The model under review builds one solid part; all positions refer to its coordinate system, in mm. Face numbers are marked on the shaded views. A direction names the side the tool comes from. Coordinates: 2 decimals unless noted, no trailing zeros. Write each loop counter-clockwise with the first axis right and the second up, starting at its lowest first coordinate (ties: lowest second). Pieces come first, ordered by that corner, then holes. Notation, with made-up numbers: M -2.75,83.25 L 48.25,83.25 A21 ccw 48.25,122.25 Z; hole C 25.25,22 d9. An arc over 180 degrees is marked long. Answer as CSV lines item,"result". Start each with the question number.
from build123d import *

# Parameters (mm, degrees)
PAD005_DEPTH           = 1
SKETCH011_R            = 2.05
POCKET008_DEPTH        = 0.32
LINEARPATTERN002_COUNT = 2
LINEARPATTERN002_PITCH = 8.7
LINEARPATTERN003_COUNT = 2
LINEARPATTERN003_PITCH = 8.7
SKETCH013_W            = 3
SKETCH013_H            = 0.75
POCKET009_DEPTH        = 0.5


with BuildPart() as part:
    # Sketch010 (on DatumPlane) → Pad005 (new body)
    with BuildSketch(Plane(origin=(0, 0, 1.2), x_dir=(1, 0, 0), z_dir=(0, 0, -1))):
        with BuildLine():
            ThreePointArc((18.55, -6.11), (14.55, -10.11), (18.55, -14.11))
            Line((18.55, -14.11), (27.25, -14.11))
            ThreePointArc((27.25, -14.11), (31.25, -10.11), (27.25, -6.11))
            Line((18.55, -6.11), (27.25, -6.11))
        make_face()
    extrude(amount=-PAD005_DEPTH)

    # Sketch011 (on Face2 of Pad005) → Pocket008 (cut)
    with BuildSketch(Plane(origin=(0, 0, 1.2), x_dir=(1, 0, 0), z_dir=(0, 0, -1))):
        with Locations((18.55, -10.11)):
            Circle(SKETCH011_R)
    pocket008 = extrude(amount=-POCKET008_DEPTH, mode=Mode.SUBTRACT)

    # LinearPattern002: Pocket008 ×2
    with Locations(*[(i * LINEARPATTERN002_PITCH, 0, 0) for i in range(1, LINEARPATTERN002_COUNT)]):
        add(pocket008, mode=Mode.SUBTRACT)

    # Sketch012 (on DatumPlane) → Revolution001 (revolve)
    with BuildSketch(Plane(origin=(18.55, 6.74, 1.2), x_dir=(0, -1, 0), z_dir=(-1, 0, 0))):
        with BuildLine():
            Line((-3.37, 1), (-3.37, 2.4))
            ThreePointArc((-0.604564, 2.25), (-1.985249, 2.362472), (-3.37, 2.4))
            ThreePointArc((-0.47, 2.1), (-0.508571, 2.200756), (-0.604564, 2.25))
            Line((-0.47, 1), (-0.47, 2.1))
            Line((-3.37, 1), (-0.47, 1))
        make_face()
    revolution001 = revolve(axis=Axis((18.55, 10.11, 1.2), (0, 0, -1)))

    # LinearPattern003: Revolution001 ×2
    with Locations(*[(i * LINEARPATTERN003_PITCH, 0, 0) for i in range(1, LINEARPATTERN003_COUNT)]):
        add(revolution001)

    # Sketch013 (on DatumPlane) → Pocket009 (cut)
    with BuildSketch(Plane(origin=(27.25, 10.11, 3.6), x_dir=(-1, 0, 0), z_dir=(0, 0, 1))):
        Polygon((1, 1.732051), (-2, 0), (1, -1.732051), align=None)
        with Locations((8.7, 0)):
            Rectangle(SKETCH013_W, SKETCH013_H)
        with Locations((8.7, 1.125)):
            Rectangle(SKETCH013_W, SKETCH013_H)
        with Locations((8.7, -1.125)):
            Rectangle(SKETCH013_W, SKETCH013_H)
    extrude(amount=-POCKET009_DEPTH, mode=Mode.SUBTRACT)


solid = part.part
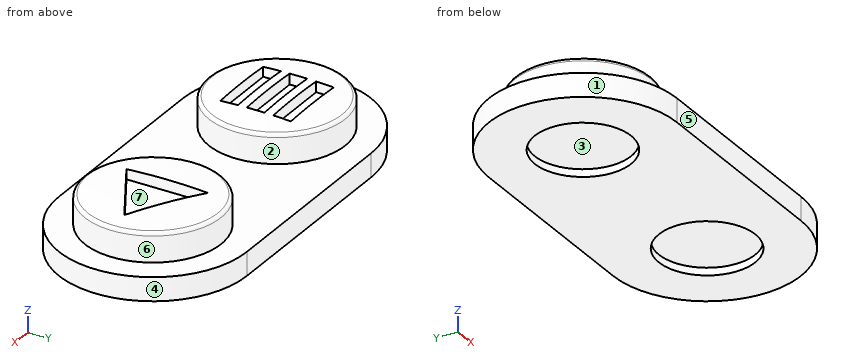
1) Take a section at A-A on z = 2.85. Give the boundary of the cut face in (x, y), and give its area (3 significant figures).
2) Tool access review of the marked faces 1, 2 and 3: name each direction out of +Z, -Z, +X, -X, +Y, -Y from which nothing blocks a thin tool from reaching the whole face with its end or side.
3) Take a section at C-C on y = 7. Give the boundary of the cut face in (x, z), and give its area (3 significant figures).
4) Take a section at B-B on x = 24. Give the boundary of the cut face in (y, z).
5) Clearance check with flat-ended pins moving along their axes: pin 1 Ø0.8 at (x, y) = (19.5, 10) entering from +Z; pin 2 Ø2.5 at (x, y) = (21.5, 11) entering from +Z; pin 3 Ø1 at (x, z) = (28, 3) entering from +Y. State where each tip first meets the part, or that it passes through.
6) To check wall thickness, follow line 1 (X direction, y = 10.11, z = 1.4); line 2 (Y direction, x = 27.25, z = 1.35); line 3 (X direction, y = 11, z = 3.2). State the ranges of each line that lie inside material, in increasing order. Write a range as [from, to].
7) Mouldability with a two-part tool opening along X and no side actions: class the marked faces 4, 5, 6 and 7 as +X half, -X half, draft (parallel to the pull), parting line (faces both ways), or undercut.
Results:
1,outline,"C 18.55,10.11 d5.8; C 27.25,10.11 d5.8"
1,area,"52.8 mm²"
2,face 1,"+Z, -Z, -X"
2,face 2,"+Z"
2,face 3,"-Z"
3,outline,"M 16.03,1.2 L 29.77,1.2 L 29.77,2.2 L 16.03,2.2 Z"
3,area,"13.7 mm²"
4,outline,"M 6.11,1.2 L 14.11,1.2 L 14.11,2.2 L 6.11,2.2 Z"
5,pin 1,"stops at z = 3.59"
5,pin 2,"stops at z = 3.53"
5,pin 3,"stops at y = 13"
6,line 1,"x = [14.55, 16.5], [20.6, 25.2], [29.3, 31.25]"
6,line 2,"y = [6.11, 8.06], [12.16, 14.11]"
6,line 3,"x = [15.79, 17.05], [20.05, 21.31], [24.49, 26.25], [27.71, 30.01]"
7,face 4,"+X half"
7,face 5,"draft"
7,face 6,"undercut"
7,face 7,"undercut"
